Job drawing, mm, ordinate dimensions from the low corner. One solid piece. A direction names the side the tool comes from. Give positions to 0.01 mm unless a question says otherwise; leave off trailing zeros. Order: outer loops, then holes, each group sorted by start corner. A loop starts at its lowest first (then second) coordinate and runs counter-clockwise, first axis right, second up.
Item 1: Band-saw the part on B-B on y = 20.5. Give the cut face in (x, z).
Item 2: Which spindle directions (+Z, -Z, +X, -X, +Y, -Y) get a long thin tool onto all of the face, cutting with end or side? Do the marked faces 1, 2 and 3. Say none if no direction does.
Item 3: Two-plate mould, pull along Y, no slides. Class the marked faces 4, 5 and 6: released by +Y, released by -Y, zero draft, split by the parting line, or undercut.
Item 4: Flat gauge pins, fed straight in: P1, Ø3.5, axis at y = 5, z = 25, coming from the -X side; P2, Ø2, axis at x = 3, z = 13, coming from the -Y side; P3, Ø5, axis at y = 5, z = 11.67, coming from the +X side. Where does each tip first touch, or does it go through?
Item 5: Wall check: L1, parallel to Z at x = 5, y = 5; L2, parallel to Y at x = 5.9, z = 5; L3, parallel to X at y = 19.75, z = 16. Give the ranges that are in metal, low to high.
Item 6: Band-saw the part on D-D on y = 5. Give the cut face in (x, z).
Item 7: Band-saw the part on C-C on x = 9.25. Give the cut face in (y, z).
Item 8: Band-saw the part on A-A on z = 5. Give the cut face in (x, y).
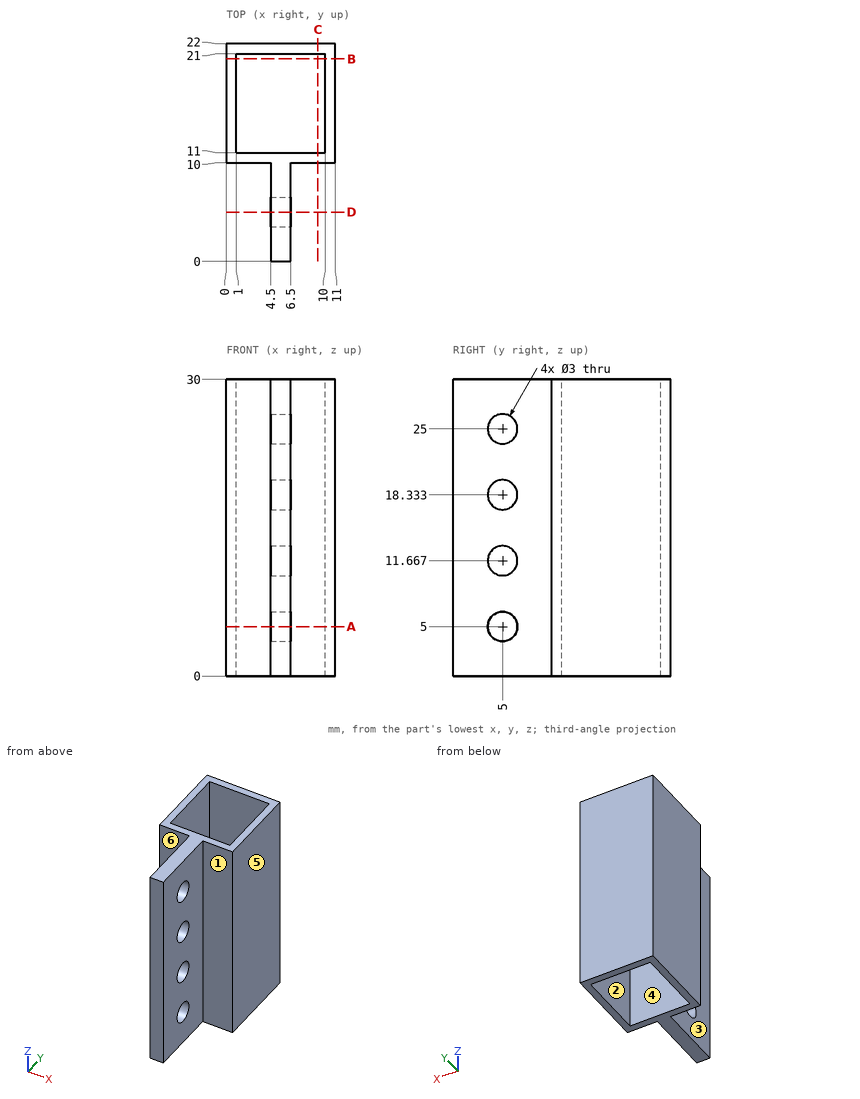
The answers:
1. outline: (0, 0) - (1, 0) - (1, 30) - (0, 30) - close; (10, 0) - (11, 0) - (11, 30) - (10, 30) - close
2. face 1: +Z, -Z, +X, -Y
2. face 2: +Z, -Z
2. face 3: +Z, -Z, -X, -Y
3. face 4: undercut
3. face 5: zero draft
3. face 6: released by -Y
4. P1: stops at x = 4.5
4. P2: stops at y = 10
4. P3: stops at x = 6.5
5. L1: z = 0 to 3.5, 6.5 to 10.17, 13.17 to 16.83, 19.83 to 23.5, 26.5 to 30
5. L2: y = 0 to 3.5, 6.5 to 11, 21 to 22
5. L3: x = 0 to 1, 10 to 11
6. outline: (4.5, 0) - (6.5, 0) - (6.5, 3.5) - (4.5, 3.5) - close; (4.5, 6.5) - (6.5, 6.5) - (6.5, 10.17) - (4.5, 10.17) - close; (4.5, 13.17) - (6.5, 13.17) - (6.5, 16.83) - (4.5, 16.83) - close; (4.5, 19.83) - (6.5, 19.83) - (6.5, 23.5) - (4.5, 23.5) - close; (4.5, 26.5) - (6.5, 26.5) - (6.5, 30) - (4.5, 30) - close
7. outline: (10, 0) - (11, 0) - (11, 30) - (10, 30) - close; (21, 0) - (22, 0) - (22, 30) - (21, 30) - close
8. outline: (0, 10) - (4.5, 10) - (4.5, 6.5) - (6.5, 6.5) - (6.5, 10) - (11, 10) - (11, 22) - (0, 22) - close; (4.5, 0) - (6.5, 0) - (6.5, 3.5) - (4.5, 3.5) - close; hole (1, 11) - (10, 11) - (10, 21) - (1, 21) - close
